```python
from build123d import *

# Parameters (mm, degrees)
SKETCH1_W           = 40
SKETCH1_H           = 60
SKETCH1_R           = 1.75
BOSS_EXTRUDE1_DEPTH = 10
SKETCH3_R           = 3
CUT_EXTRUDE1_DEPTH  = 5


with BuildPart() as part:
    # Sketch1 → Boss-Extrude1 (new body)
    with BuildSketch(Plane.XY):
        Rectangle(SKETCH1_W, SKETCH1_H)
        with Locations((-16, 26)):
            Circle(SKETCH1_R, mode=Mode.SUBTRACT)
        with Locations((16, 26)):
            Circle(SKETCH1_R, mode=Mode.SUBTRACT)
        with Locations((16, -26)):
            Circle(SKETCH1_R, mode=Mode.SUBTRACT)
        with Locations((-16, -26)):
            Circle(SKETCH1_R, mode=Mode.SUBTRACT)
    extrude(amount=BOSS_EXTRUDE1_DEPTH)

    # Sketch3 → Cut-Extrude1 (cut)
    with BuildSketch(Plane.XY):
        with Locations((16, 26)):
            Circle(SKETCH3_R)
        with Locations((-16, 26)):
            Circle(SKETCH3_R)
        with Locations((16, -26)):
            Circle(SKETCH3_R)
        with Locations((-16, -26)):
            Circle(SKETCH3_R)
    extrude(amount=CUT_EXTRUDE1_DEPTH, mode=Mode.SUBTRACT)


solid = part.part
```
CAD build for the part. Positions are in the model's coordinates, mm. A direction names the side the tool comes from. Round coordinates to 2 decimals unless told otherwise and drop trailing zeros. Order: outer loops, then holes, each group sorted by start corner. A loop starts at its lowest first (then second) coordinate and runs counter-clockwise, first axis right, second up. Notation, with made-up numbers: (86.25, 23.25) -> (114.25, 23.25) arc R28 ccw to (114.25, 50.25) -> close; hole circle Ø1 at (56, 62.25). An arc over 180 degrees is marked (long way). One line per question, with ' | ' between items.
Q1. Slice it at D-D (z = 6). Write the cut outline in (x, y).
Completed:
outline: (-20, -30) -> (20, -30) -> (20, 30) -> (-20, 30) -> close; hole circle Ø3.5 at (-16, -26); hole circle Ø3.5 at (-16, 26); hole circle Ø3.5 at (16, -26); hole circle Ø3.5 at (16, 26)
Q2. Drop a flat-ended pin along its axis: pin 1 (4 mm diameter, centred on x = -16, y = -26, fed in from -Z). Give the stop position or say it passes through.
Completed:
pin 1: stops at z = 5
Q3. Probe probe 1 along Y at (x, z) = (-16, 1.9); probe 2 along Y at (x, z) = (16, 6.75); probe 3 along X at (y, z) = (-26, 7.1). List the from-to ranges inside material, lowest first.
Completed:
probe 1: y = -30 to -29, -23 to 23, 29 to 30 | probe 2: y = -30 to -27.75, -24.25 to 24.25, 27.75 to 30 | probe 3: x = -20 to -17.75, -14.25 to 14.25, 17.75 to 20
Q4. Slice it at B-B (y = -26). Write the cut outline in (x, z).
Completed:
outline: (-20, 0) -> (-19, 0) -> (-19, 5) -> (-17.75, 5) -> (-17.75, 10) -> (-20, 10) -> close; (-14.25, 5) -> (-13, 5) -> (-13, 0) -> (13, 0) -> (13, 5) -> (14.25, 5) -> (14.25, 10) -> (-14.25, 10) -> close; (17.75, 5) -> (19, 5) -> (19, 0) -> (20, 0) -> (20, 10) -> (17.75, 10) -> close
Q5. Slice it at C-C (z = 2). Write the cut outline in (x, y).
Completed:
outline: (-20, -30) -> (20, -30) -> (20, 30) -> (-20, 30) -> close; hole circle Ø6 at (-16, -26); hole circle Ø6 at (-16, 26); hole circle Ø6 at (16, -26); hole circle Ø6 at (16, 26)
Q6. Two-plate mould, pull along X, no slides. Class faces 3 (the flat face through (0, 0, 10)), 4 (the flat face through (20, 0, 5)), 5 (the cylindrical face through (15.772, -24.265, 7.465)): released by +X, released by -X, zero draft, split by the parting line, or undercut.
Completed:
face 3: zero draft | face 4: released by +X | face 5: undercut
Q7. Which spindle directions (+Z, -Z, +X, -X, +Y, -Y) get a long thin tool onto all of the face, cutting with end or side? Do faces 1 (the cylindrical face through (15.772, 27.735, 7.465)), 2 (the flat face through (18, 26, 5)). Say none if no direction does.
Completed:
face 1: +Z, -Z | face 2: -Z
Q8. Slice it at A-A (x = -16). Write the cut outline in (y, z), then the cut area to 3 significant figures.
Completed:
outline: (-30, 0) -> (-29, 0) -> (-29, 5) -> (-27.75, 5) -> (-27.75, 10) -> (-30, 10) -> close; (-24.25, 5) -> (-23, 5) -> (-23, 0) -> (23, 0) -> (23, 5) -> (24.25, 5) -> (24.25, 10) -> (-24.25, 10) -> close; (27.75, 5) -> (29, 5) -> (29, 0) -> (30, 0) -> (30, 10) -> (27.75, 10) -> close | area: 505 mm^2
